Verification items for the finished model (mm, model axes). Face numbers are marked on the shaded views. A direction names the side the tool comes from. Round coordinates to 2 decimals unless told otherwise and drop trailing zeros. Loops run counter-clockwise (first coordinate to the right, second up) from the corner with the lowest first, then second, coordinate; pieces in that order, holes last. Notation, with made-up numbers: (-32, 5) -> (2, 5) arc R11 cw to (2, 11) -> close; hole circle Ø11 at (78.5, 47). An arc over 180 degrees is marked (long way). Write item = value, one per line. Start each with the question number.
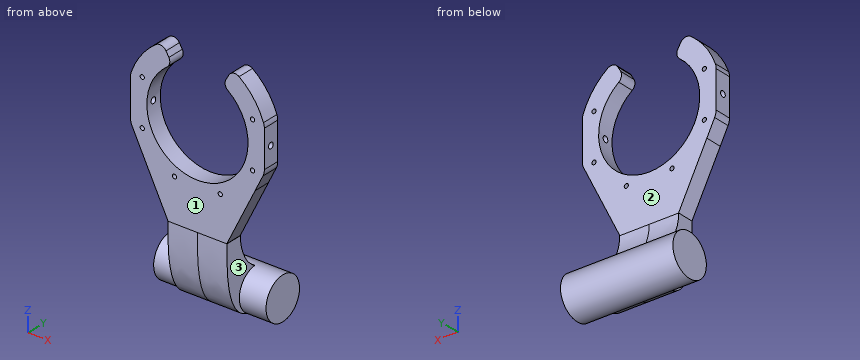
```python
from build123d import *

# Parameters (mm, degrees)
BOSS_EXTRUDE1_DEPTH = 12
SKETCH2_R           = 18
CUT_EXTRUDE1_DEPTH  = 12
BOSS_EXTRUDE2_DEPTH = 21
SKETCH8_R           = 15
BOSS_EXTRUDE4_DEPTH = 40
SKETCH12_R          = 1.5
CUT_EXTRUDE3_DEPTH  = 136.830697271
SKETCH13_R          = 36
CUT_EXTRUDE4_DEPTH  = 136.830697271
CUT_EXTRUDE5_DEPTH  = 136.830697271
FILLET1_R           = 5
M5_TAPPED_HOLE1_D   = 4.2
CUT_EXTRUDE6_DEPTH  = 136.830697306
FILLET2_R           = 10


with BuildPart() as part:
    # Sketch1 → Boss-Extrude1 (new body)
    with BuildSketch(Plane(origin=(0, 0, 0), x_dir=(1, 0, 0), z_dir=(0, 1, 0))):
        with BuildLine():
            Line((-20.882573235, 69.325415808), (20.882573235, 69.325415808))
            Line((20.882573235, 69.325415808), (41.057018878, 28.536313722))
            ThreePointArc((41.057018878, 28.536313722), (44.846867978, 22.107881683), (47.637749602, 15.186994859))
            Line((47.637749602, 15.186994859), (47.637749602, -15.186994859))
            ThreePointArc((47.637749602, -15.186994859), (0, -50), (-47.637749602, -15.186994859))
            Line((-47.637749602, -15.186994859), (-47.637749602, 15.186994859))
            ThreePointArc((-47.637749602, 15.186994859), (-44.846867978, 22.107881683), (-41.057018878, 28.536313722))
            Line((-41.057018878, 28.536313722), (-20.882573235, 69.325415808))
        make_face()
    extrude(amount=BOSS_EXTRUDE1_DEPTH)

    # Sketch2 → Cut-Extrude1 (cut)
    with BuildSketch(Plane.XZ):
        with Locations(Location((0, 0, 0), (0, 0, 270))):
            Circle(SKETCH2_R)
    extrude(amount=-CUT_EXTRUDE1_DEPTH, mode=Mode.SUBTRACT)

    # Sketch4 → Boss-Extrude2 (add, symmetric)
    with BuildSketch(Plane(origin=(0, 0, 0), x_dir=(0, 0, -1), z_dir=(1, 0, 0))):
        with BuildLine():
            add(Edge.make_bspline(
                [(69.325415808, 12), (78.050182199, 12), (89.075370915, 16.109716253), (93.862821874, 25.051459816)],
                knots=[0, 0, 0, 0, 0.77117819, 0.77117819, 0.77117819, 0.77117819], degree=3))
            Line((69.325415808, 12), (69.325415808, 0))
            add(Edge.make_bspline(
                [(69.325415808, 0), (85.617905629, 0), (116.367065239, -0.702532384), (121.3953127, 17.938299278)],
                knots=[0, 0, 0, 0, 1, 1, 1, 1], degree=3))
            ThreePointArc((121.3953127, 17.938299278), (105.072430052, 11.59905464), (93.862821874, 25.051459816))
        make_face()
    extrude(amount=BOSS_EXTRUDE2_DEPTH, both=True)

    # Sketch8 → Boss-Extrude4 (add, symmetric)
    with BuildSketch(Plane(origin=(0, 0, 0), x_dir=(0, 0, -1), z_dir=(1, 0, 0))):
        with Locations((108.824557436, 26.122192734)):
            Circle(SKETCH8_R)
    extrude(amount=BOSS_EXTRUDE4_DEPTH, both=True)

    # Sketch12 → Cut-Extrude3 (cut, through all)
    with BuildSketch(Plane(origin=(0, 12, 0), x_dir=(1, 0, 0), z_dir=(0, 1, 0))):
        with Locations(Location((-16.264045876, 39.264880132, 0), (0, 0, 270))):
            Circle(SKETCH12_R)
        with Locations(Location((16.264045876, 39.264880132, 0), (0, 0, 270))):
            Circle(SKETCH12_R)
        with Locations(Location((39.264880132, 16.264045876, 0), (0, 0, 270))):
            Circle(SKETCH12_R)
        with Locations(Location((39.264880132, -16.264045876, 0), (0, 0, 270))):
            Circle(SKETCH12_R)
        with Locations(Location((-39.264880132, -16.264045876, 0), (0, 0, 270))):
            Circle(SKETCH12_R)
        with Locations(Location((-39.264880132, 16.264045876, 0), (0, 0, 270))):
            Circle(SKETCH12_R)
    extrude(amount=-CUT_EXTRUDE3_DEPTH, mode=Mode.SUBTRACT)

    # Sketch13 → Cut-Extrude4 (cut, through all)
    with BuildSketch(Plane(origin=(0, 12, 0), x_dir=(1, 0, 0), z_dir=(0, 1, 0))):
        with Locations(Location((0, 0, 0), (0, 0, 270))):
            Circle(SKETCH13_R)
    extrude(amount=-CUT_EXTRUDE4_DEPTH, mode=Mode.SUBTRACT)

    # Sketch14 → Cut-Extrude5 (cut, through all)
    with BuildSketch(Plane(origin=(0, 12, 0), x_dir=(1, 0, 0), z_dir=(0, 1, 0))):
        with BuildLine():
            Line((0, 0), (-48.782083041, -84.493046326))
            ThreePointArc((-48.782083041, -84.493046326), (0, -97.564166081), (48.782083041, -84.493046326))
            Line((48.782083041, -84.493046326), (0, 0))
        make_face()
    extrude(amount=-CUT_EXTRUDE5_DEPTH, mode=Mode.SUBTRACT)

    # Fillet1
    fillet1_edges = [part.edges().sort_by_distance(p)[0] for p in [
        (-18, 6, 31.176914536),
        (18, 6, 31.176914536),
        (25, 6, 43.301270189),
        (-25, 6, 43.301270189),
    ]]
    fillet(fillet1_edges, radius=FILLET1_R)

    # M5 Tapped Hole1 (through all)
    with Locations(Plane(origin=(-47.637749602, 5.86539704, 5.141e-06), x_dir=(0, 0, -1), z_dir=(-1, 0, 0))):
        with Locations((0, 0)):
            Hole(M5_TAPPED_HOLE1_D / 2)

    # Sketch30 → Cut-Extrude6 (cut, through all)
    with BuildSketch(Plane(origin=(0, 12, 0), x_dir=(1, 0, 0), z_dir=(0, 1, 0))):
        Polygon((-41.057018878, 28.536313722), (-47.637749602, 15.186994859), (-55.094112821, 25.321901869), align=None)
        Polygon((41.057018878, 28.536313722), (47.637749602, 15.186994859), (61.944517535, 29.154568453), align=None)
    extrude(amount=-CUT_EXTRUDE6_DEPTH, mode=Mode.SUBTRACT)

    # Fillet2
    fillet2_edges = [part.edges().sort_by_distance(p)[0] for p in [
        (-41.057018878, 6, -28.536313722),
        (41.057018878, 6, -28.536313722),
        (47.637749602, 6, -15.186994859),
        (47.637749602, 6, 15.186994859),
        (-47.637749602, 6, 15.186994859),
        (-47.637749602, 6, -15.186994859),
    ]]
    fillet(fillet2_edges, radius=FILLET2_R)


solid = part.part
```
(1) Section check C-C on z = 31.5. Enter the section's corners in (x, y), then the cut area to 3 significant figures.
(2) Scan lines: line 1 (X direction, y = 2.5, z = 0); line 2 (X direction, y = 10, z = -105); line 3 (Y direction, x = 26.5, z = -36.5). Record each from-to range of solid material in increasing order. Write a range as [from, to].
(3) Depth check by flat-ended pin: pin 1 Ø3.5 at (x, z) = (-39.26, -16.26) entering from -Y; pin 2 Ø7.5 at (y, z) = (10.5, -90) entering from -X; pin 3 Ø3 at (y, z) = (19, -105) entering from -X. Enter the tip coordinate at first touch or a pass-through.
(4) Section check B-B on x = 26. Enter the section's corners in (y, z), then the cut area to 3 significant figures.
(5) Access from +Z, -Z, +X, -X, +Y, -Y to the whole of each face (thin tool, end or side, straight path). Record for the marked faces 1, 2 and 3.
(6) Section check A-A on z = 0. Enter the section's corners in (x, y).
(7) Section check D-D on y = 35.5. Enter the section's corners in (x, z).
Computed values:
q1.outline = (-38.83, 0) -> (-19.83, 0) -> (-19.83, 12) -> (-38.83, 12) -> close; (19.83, 0) -> (38.83, 0) -> (38.83, 12) -> (19.83, 12) -> close
q1.area = 456 mm²
q2.line_1 = [-47.64, -36], [36, 47.64]
q2.line_2 = [-21, 21]
q2.line_3 = [0, 12]
q3.pin_1 = 0
q3.pin_2 = -21
q3.pin_3 = -40
q4.outline = (0, -58.98) -> (12, -58.98) -> (12, -24.9) -> (0, -24.9) -> close; (0, 24.9) -> (12, 24.9) -> (12, 41.18) -> (0, 41.18) -> close; circle Ø30 at (26.12, -108.82)
q4.area = 1,310 mm²
q5.face_1 = +Z, -Z, +X, -X, -Y
q5.face_2 = +Z, +X, -X, +Y
q5.face_3 = +X, -Y
q6.outline = (-47.64, 0) -> (-36, 0) -> (-36, 3.77) -> (-47.64, 3.77) -> close; (-47.64, 7.97) -> (-36, 7.97) -> (-36, 12) -> (-47.64, 12) -> close; (36, 0) -> (47.64, 0) -> (47.64, 3.77) -> (36, 3.77) -> close; (36, 7.97) -> (47.64, 7.97) -> (47.64, 12) -> (36, 12) -> close
q7.outline = (-40, -120.53) -> (40, -120.53) -> (40, -97.12) -> (-40, -97.12) -> close
